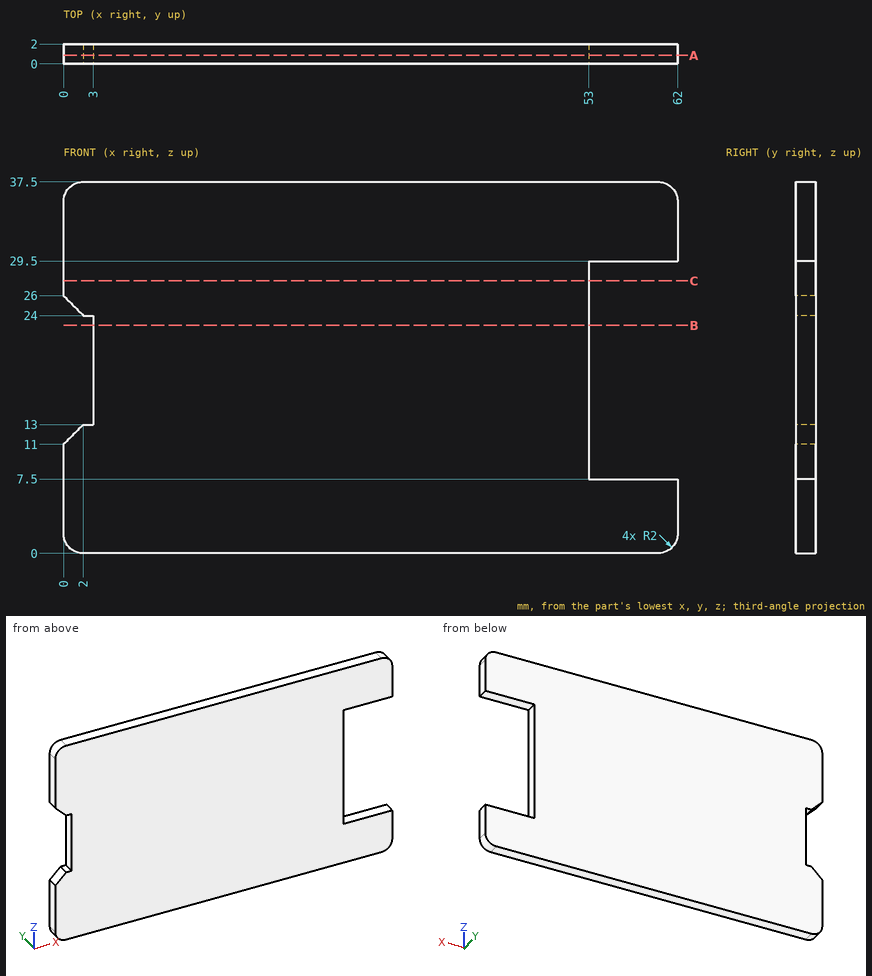
Could you check a few things on this drawing? It's one solid part, dimensions in mm from its lowest x, y, z. Coordinates: 2 decimals unless noted, no trailing zeros. Write each loop counter-clockwise with the first axis right and the second up, starting at its lowest first coordinate (ties: lowest second). Pieces come first, ordered by that corner, then holes.
Q1. Please list where these lines run through material, in increasing order: L1, parallel to X at y = 1.35, z = 23.5; L2, parallel to X at y = 0.3, z = 28.5.
Results found:
L1: x = 3 to 53
L2: x = 0 to 53
Q2. Imagine slicing it at B-B, the plane z = 23. List the corners of the cut face in (x, y) for me, plus the area to 3 significant figures.
Results found:
outline: (3, 0) - (53, 0) - (53, 2) - (3, 2) - close
area: 100 mm2
Q3. Imagine slicing it at A-A, the plane y = 0.85. List the corners of the cut face in (x, z) for me.
Results found:
outline: (0, 2) arc R2 ccw to (2, 0) - (60, 0) arc R2 ccw to (62, 2) - (62, 7.5) - (53, 7.5) - (53, 29.5) - (62, 29.5) - (62, 35.5) arc R2 ccw to (60, 37.5) - (2, 37.5) arc R2 ccw to (0, 35.5) - (0, 26) - (2, 24) - (3, 24) - (3, 13) - (2, 13) - (0, 11) - close
Q4. Imagine slicing it at C-C, the plane z = 27.5. List the corners of the cut face in (x, y) for me, plus the area to 3 significant figures.
Results found:
outline: (0, 0) - (53, 0) - (53, 2) - (0, 2) - close
area: 106 mm2
Q5. For P1, Ø1, axis at y = 0.5, z = 16.5, coming from the -X side; P2, Ø3, axis at x = 55.5, z = 10, coming from the -Y side, each with a flat end and sliding along its axis, tell me the tip position at first contact or that it passes through.
Results found:
P1: stops at x = 3
P2: passes through
